Job drawing, mm, ordinate dimensions from the low corner. One solid piece. A direction names the side the tool comes from. Give positions to 0.01 mm unless a question says otherwise; leave off trailing zeros. Loops run counter-clockwise (first coordinate to the right, second up) from the corner with the lowest first, then second, coordinate; pieces in that order, holes last. Notation, with made-up numbers: (-33.5, 82.5) -> (-18.5, 82.5) arc R9 cw to (-18.5, 90.5) -> close; hole circle Ø5 at (5, -13.75). An arc over 180 degrees is marked (long way). Use one line per item in the form item = value.
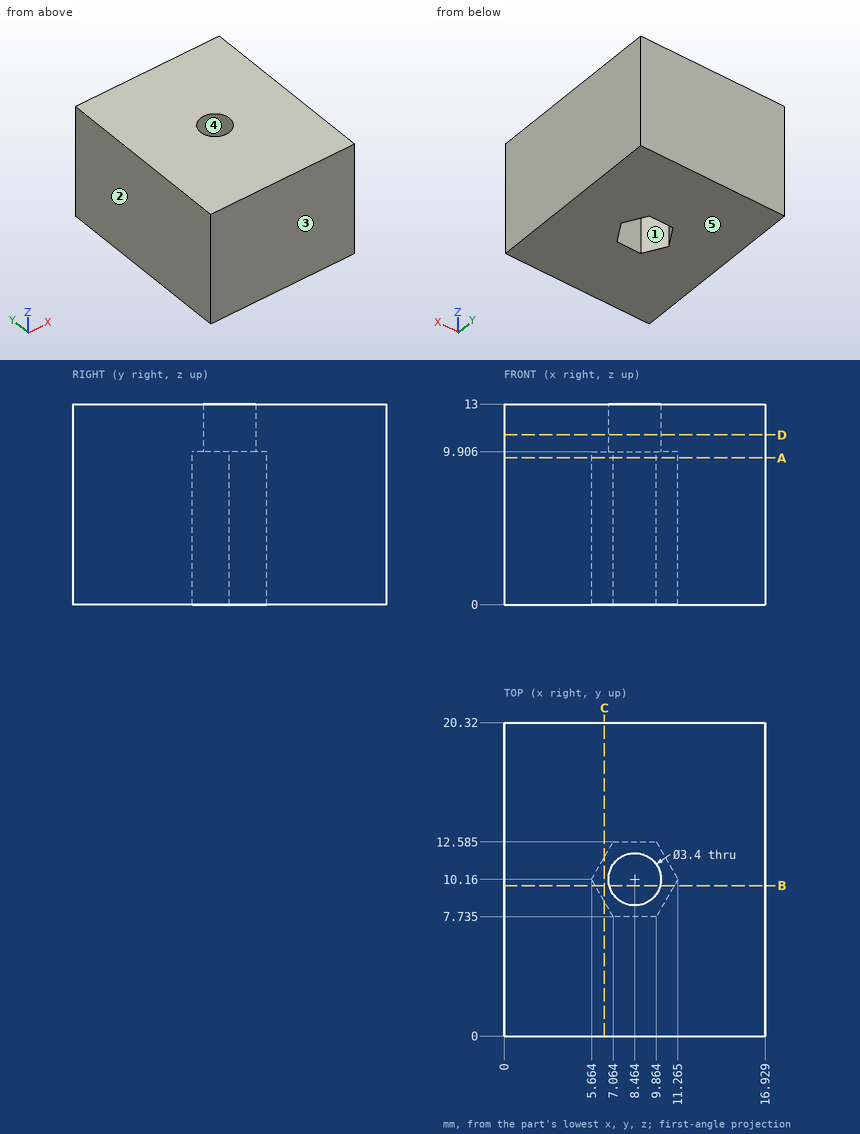
1. Tool access for the marked faces 1 and 2: list every direction of +Z, -Z, +X, -X, +Y, -Y with a clear straight run to the whole face (end or side of a thin tool).
Result sheet:
face_1 = -Z
face_2 = +Z, -Z, -X, +Y, -Y
2. Cut at A-A, the plane z = 9.5. Write the cut outline in (x, y) (1 decimal), then the cut area to 3 significant figures.
Result sheet:
outline = (0, 0) -> (16.9, 0) -> (16.9, 20.3) -> (0, 20.3) -> close; hole (5.7, 10.2) -> (7.1, 7.7) -> (9.9, 7.7) -> (11.3, 10.2) -> (9.9, 12.6) -> (7.1, 12.6) -> close
area = 324 mm^2
3. Cut at C-C, the plane x = 6.5. Write the cut outline in (y, z).
Result sheet:
outline = (0, 0) -> (8.71, 0) -> (8.71, 9.91) -> (11.61, 9.91) -> (11.61, 0) -> (20.32, 0) -> (20.32, 13) -> (0, 13) -> close
4. Cut at B-B, the plane y = 9.75. Write the cut outline in (x, z) (1 decimal).
Result sheet:
outline = (0, 0) -> (5.9, 0) -> (5.9, 9.9) -> (6.8, 9.9) -> (6.8, 13) -> (0, 13) -> close; (10.1, 9.9) -> (11, 9.9) -> (11, 0) -> (16.9, 0) -> (16.9, 13) -> (10.1, 13) -> close
5. Drill centre lines: line 1 (Y direction, x = 9, z = 6) (1 decimal); line 2 (Z direction, x = 10.25, y = 9.75); line 3 (X direction, y = 10.5, z = 7.75). Where is each one in solid material? Low to high.
Result sheet:
line_1 = 0 to 7.7, 12.6 to 20.3
line_2 = 9.91 to 13
line_3 = 0 to 5.86, 11.07 to 16.93
6. Cut at D-D, the plane z = 11. Write the cut outline in (x, y) (1 decimal), then the cut area to 3 significant figures.
Result sheet:
outline = (0, 0) -> (16.9, 0) -> (16.9, 20.3) -> (0, 20.3) -> close; hole circle Ø3.4 at (8.5, 10.2)
area = 335 mm^2
7. Mould opens along Y. For the marked faces 3, 4 and 5 say: pulls with the +Y half, pulls with the -Y half, needs draft (parallel to the pull), parting line crosses it, or undercut.
Result sheet:
face_3 = pulls with the -Y half
face_4 = undercut
face_5 = needs draft
